The listing builds one solid part. Answer for the finished solid, in the listing's coordinates (mm). A direction names the side the tool comes from. Round coordinates to 2 decimals unless told otherwise and drop trailing zeros. Write each loop counter-clockwise with the first axis right and the second up, starting at its lowest first coordinate (ties: lowest second). Pieces come first, ordered by that corner, then holes. Notation, with made-up numbers: M 76.25,-6.5 L 102.25,-6.5 A33 ccw 102.25,28.5 Z; hole C 75,-33.5 d7. An arc over 180 degrees is marked long. Write each question's results on one line, items separated by ' | '.
from build123d import *

# Parameters (mm, degrees)
SKETCH1_R           = 19
SKETCH1_R_2         = 2.5
SKETCH1_R_3         = 8
BOSS_EXTRUDE1_DEPTH = 3
SKETCH1_5_R         = 19
SKETCH1_5_R_2       = 18
BOSS_EXTRUDE2_DEPTH = 90
SKETCH2_R           = 5.25
CUT_EXTRUDE1_DEPTH  = 20


with BuildPart() as part:
    # Sketch1 → Boss-Extrude1 (new body)
    with BuildSketch(Plane(origin=(0, 0, 0), x_dir=(1, 0, 0), z_dir=(0, 1, 0))):
        Circle(SKETCH1_R)
        with Locations((-13.05625, 0)):
            Circle(SKETCH1_R_2, mode=Mode.SUBTRACT)
        Circle(SKETCH1_R_3, mode=Mode.SUBTRACT)
    extrude(amount=BOSS_EXTRUDE1_DEPTH)

    # Sketch1_5 → Boss-Extrude2 (add)
    with BuildSketch(Plane(origin=(0, 0, 0), x_dir=(1, 0, 0), z_dir=(0, 1, 0))):
        Circle(SKETCH1_5_R)
        Circle(SKETCH1_5_R_2, mode=Mode.SUBTRACT)
    extrude(amount=BOSS_EXTRUDE2_DEPTH)

    # Sketch2 → Cut-Extrude1 (cut, through all)
    with BuildSketch(Plane(origin=(0, 0, 0), x_dir=(0, 0, -1), z_dir=(1, 0, 0))):
        with Locations((0, 17)):
            Circle(SKETCH2_R)
    extrude(amount=-CUT_EXTRUDE1_DEPTH, mode=Mode.SUBTRACT)


solid = part.part
1) Section B-B (z = 0) is taken. Determine the outline of the cut face in (x, y).
Return value:
outline: M -19,0 L -15.56,0 L -15.56,3 L -18,3 L -18,11.75 L -19,11.75 Z; M -19,22.25 L -18,22.25 L -18,90 L -19,90 Z; M -10.56,0 L -8,0 L -8,3 L -10.56,3 Z; M 8,0 L 19,0 L 19,90 L 18,90 L 18,3 L 8,3 Z
2) Section C-C (z = 6.5) is taken. Determine the outline of the cut face in (x, y), then the cut area to 3 significant figures.
Return value:
outline: M -17.85,0 L -4.66,0 L -4.66,3 L -16.79,3 L -16.79,90 L -17.85,90 Z; M 4.66,0 L 17.85,0 L 17.85,90 L 16.79,90 L 16.79,3 L 4.66,3 Z | area: 265 mm²
3) The mould has two halves that part along X. Classify faces 1 (the face through (17.55, 44.37, 7.28)), 2 (the face through (8, 3, 4)), 3 (the face through (7, 90, 17)): +X half, -X half, draft (parallel to the pull), parting line (faces both ways), or undercut.
Return value:
face 1: parting line | face 2: undercut | face 3: draft
4) Find the intervals of material crossed by line 1 (X direction, y = 0.9, z = 0); line 2 (Y direction, x = -18.25, z = 0); line 3 (Z direction, x = 0, y = 20), in increasing order.
Return value:
line 1: -19 to -15.56, -10.56 to -8, 8 to 19 | line 2: 0 to 11.75, 22.25 to 90 | line 3: -19 to -18, 18 to 19
5) Section D-D (x = 16) is taken. Determine the outline of the cut face in (y, z), then the cut area to 3 significant figures.
Return value:
outline: M 0,-10.25 L 90,-10.25 L 90,-8.25 L 3,-8.25 L 3,8.25 L 90,8.25 L 90,10.25 L 0,10.25 Z | area: 410 mm²
6) Section A-A (x = 0) is taken. Determine the outline of the cut face in (y, z), then the cut area to 3 significant figures.
Return value:
outline: M 0,-19 L 90,-19 L 90,-18 L 3,-18 L 3,-8 L 0,-8 Z; M 0,8 L 3,8 L 3,18 L 90,18 L 90,19 L 0,19 Z | area: 240 mm²
7) A tool of negligible diameter and unlimited length cuts with its end or side. For faces 4 (the face through (17.169, 45.891, -5.407)), 5 (the face through (-1.73, 1.48, 7.81)), 6 (the face through (-18.1, 18.6, -5)), from which of +Z, -Z, +X, -X, +Y, -Y can it reach the whole face along a straight path? Write none if from no direction.
Return value:
face 4: +Y | face 5: +Y, -Y | face 6: -X
8) Each of these flat-tipped pins is pushed along its axis until it touches: pin 1 (8 mm diameter, centred on y = 44.5, z = -11.5, fed in from +X); pin 2 (5 mm diameter, centred on x = 2, y = 68, fed in from -Z); pin 3 (2 mm diameter, centred on x = 10.5, y = 59, fed in from -Z). Where does it stop, or does it pass through?
Return value:
pin 1: x = 17.46 | pin 2: z = -19 | pin 3: z = -16.45
